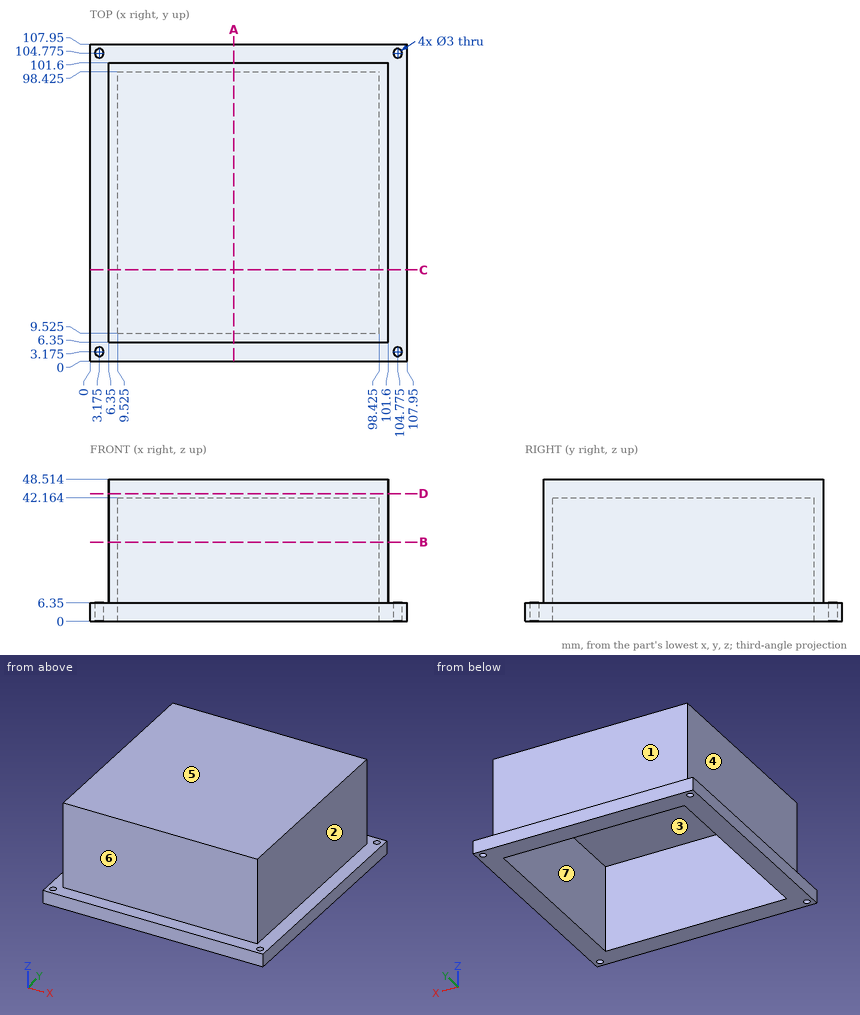
Can you work these out from the drawing? Everything is in mm from the part's minimum corner. A direction names the side the tool comes from. Give positions to 0.01 mm unless a question says otherwise; leave off trailing zeros. Order: outer loops, then holes, each group sorted by start corner. A loop starts at its lowest first (then second) coordinate and runs counter-clockwise, first axis right, second up. Notation, with made-up numbers: M 14,35.25 L 64,35.25 A14 ccw 64,60.25 Z; hole C 78,25 d11. An arc over 180 degrees is marked long. Write item = value, one per line. Start each with the question number.
Q1. We'd pull the mould along X, two halves only. Please class the marked faces 1, 2, 3 and 4: pulls with the +X half, pulls with the -X half, needs draft (parallel to the pull), parting line crosses it, or undercut.
Q2. Suppose I cut it at A-A (x = 49). Write out the boundary of the cut face in (y, z) (3 decimals).
Q3. For the marked faces 5, 6 and 7, which set-ups out of +Z, -Z, +X, -X, +Y, -Y let a thin tool reach every point of the face, with its end or its side?
Q4. Will these pins go through, and if not, where does the flat tip stop? pin 1 Ø1.5 at (y, z) = (13, 32.5) entering from -X; pin 2 Ø3 at (x, y) = (85, 15.5) entering from -Z; pin 3 Ø2.5 at (x, y) = (3.175, 104.775) entering from +Z; pin 4 Ø2 at (x, z) = (35, 40) entering from +Y.
Q5. Suppose I cut it at D-D (z = 43.5). Write out the boundary of the cut face in (x, y).
Q6. I need wall thicknesses on probe 1 along X at (y, z) = (79.5, 37) (3 decimals); probe 2 along Y at (x, z) = (44.5, 5) (3 decimals). Which ranges of each line are inside material? Lowest first, please. Write a range as [from, to].
Q7. Suppose I cut it at B-B (z = 27). Write out the boundary of the cut face in (x, y) (3 decimals), plus the area to 3 significant figures.
Check result:
q1.face_1 = needs draft
q1.face_2 = pulls with the +X half
q1.face_3 = undercut
q1.face_4 = pulls with the -X half
q2.outline = M 0,0 L 9.525,0 L 9.525,42.164 L 98.425,42.164 L 98.425,0 L 107.95,0 L 107.95,6.35 L 101.6,6.35 L 101.6,48.514 L 6.35,48.514 L 6.35,6.35 L 0,6.35 Z
q3.face_5 = +Z, +X, -X, +Y, -Y
q3.face_6 = +Z, +X, -X, -Y
q3.face_7 = -Z
q4.pin_1 = 6.35
q4.pin_2 = 42.16
q4.pin_3 = through
q4.pin_4 = 101.6
q5.outline = M 6.35,6.35 L 101.6,6.35 L 101.6,101.6 L 6.35,101.6 Z
q6.probe_1 = [6.35, 9.525], [98.425, 101.6]
q6.probe_2 = [0, 9.525], [98.425, 107.95]
q7.outline = M 6.35,6.35 L 101.6,6.35 L 101.6,101.6 L 6.35,101.6 Z; hole M 9.525,9.525 L 98.425,9.525 L 98.425,98.425 L 9.525,98.425 Z
q7.area = 1,170 mm2
